```python
from build123d import *

# Parameters (mm, degrees)
SKETCH2_R           = 22.225
SKETCH2_R_2         = 19.05
SKETCH2_R_3         = 15.875
BOSS_EXTRUDE1_DEPTH = 3.175
SKETCH3_R           = 1.5875
BOSS_EXTRUDE2_DEPTH = 3.175
CUT_EXTRUDE1_DEPTH  = 3.175


with BuildPart() as part:
    # Sketch2 → Boss-Extrude1 (new body)
    with BuildSketch(Plane.XY):
        Circle(SKETCH2_R)
        Circle(SKETCH2_R_2, mode=Mode.SUBTRACT)
        Circle(SKETCH2_R_2)
        Circle(SKETCH2_R_3, mode=Mode.SUBTRACT)
    extrude(amount=BOSS_EXTRUDE1_DEPTH)

    # Sketch3 → Boss-Extrude2 (add)
    with BuildSketch(Plane.XY.offset(3.175)):
        with BuildLine():
            ThreePointArc((-16.148535057, 15.270083186), (-13.77482484, 17.441468562), (-11.1125, 19.247414599))
            Line((-11.1125, 19.247414599), (-17.4625, 30.245937227))
            Line((-17.4625, 30.245937227), (-22.961761314, 27.070937227))
            Line((-22.961761314, 27.070937227), (-16.611761314, 16.072414599))
            Line((-16.611761314, 16.072414599), (-16.148535057, 15.270083186))
        make_face()
        with Locations((-18.624630657, 25.90880657)):
            Circle(SKETCH3_R, mode=Mode.SUBTRACT)
        with BuildLine():
            Line((17.4625, 30.245937227), (11.1125, 19.247414599))
            ThreePointArc((11.1125, 19.247414599), (13.77482484, 17.441468562), (16.148535057, 15.270083186))
            Line((16.148535057, 15.270083186), (16.611761314, 16.072414599))
            Line((16.611761314, 16.072414599), (22.961761314, 27.070937227))
            Line((22.961761314, 27.070937227), (17.4625, 30.245937227))
        make_face()
        with Locations((18.624630657, 25.90880657)):
            Circle(SKETCH3_R, mode=Mode.SUBTRACT)
    extrude(amount=-BOSS_EXTRUDE2_DEPTH)

    # Sketch5 → Cut-Extrude1 (cut)
    with BuildSketch(Plane.XY.offset(3.175)):
        with BuildLine():
            Line((-11.1125, 19.247414599), (0, 0))
            Line((0, 0), (11.1125, 19.247414599))
            ThreePointArc((11.1125, 19.247414599), (0, 22.225), (-11.1125, 19.247414599))
        make_face()
    extrude(amount=-CUT_EXTRUDE1_DEPTH, mode=Mode.SUBTRACT)


solid = part.part
```
Could you check a few things on this model? Use its own coordinates, in mm. A direction names the side the tool comes from. Round coordinates to 2 decimals unless told otherwise and drop trailing zeros. Order: outer loops, then holes, each group sorted by start corner. A loop starts at its lowest first (then second) coordinate and runs counter-clockwise, first axis right, second up. Notation, with made-up numbers: M -27,-35.5 L -19,-35.5 A16 cw -19,-13.5 Z; hole C 24.5,57.5 d6. An arc over 180 degrees is marked long. One line per question, with ' | ' between items. Start each with the question number.
(1) Please list where these lines run through material, in increasing order: line 1 along X through (y, z) = (0, 1.95) (3 decimals); line 2 along Y through (x, z) = (18, 0.5); line 3 along X through (y, z) = (7, 2.3).
(2) Suppose I cut it at B-B on z = 1.75. Count the separate pieces of the cut face and the enclosed holes in it, then the cut area to 3 significant figures.
(3) For faces 1 (the face through (-12.633, 21.882, 1.61)), 2 (the face through (-20.174, 28.681, 1.61)), which set-ups out of +Z, -Z, +X, -X, +Y, -Y let a thin tool reach every point of the face, with its end or its side?
(4) For P1, Ø1, axis at y = -1, z = 1, coming from the +X side; P2, Ø1, axis at y = 7.5, z = 2.5, coming from the -X side, each with a flat end and sliding along its axis, tell me the tip position at first contact or that it passes through.
(5) Thinking about a two-plate mould opening in Y: for faces 3 (the face through (12.633, 21.882, 1.61)), 4 (the face through (-17.89, 24.5, 1.61)), 5 (the face through (-9, 14, 3.175)), 6 (the face through (19.36, 24.5, 1.61)), which applies, +Y half, -Y half, draft (parallel to the pull), parting line (faces both ways), or undercut?
(6) Suppose I cut it at C-C on x = 12. List the corners of the cut face in (y, z) for me (3 decimals), then the cut area to 3 significant figures.
(7) Suppose I cut it at A-A on y = 4. List the corners of the cut face in (x, z) for me (3 decimals), then the cut area to 3 significant figures.
(8) Suppose I cut it at D-D on x = 0. List the corners of the cut face in (y, z) for me (3 decimals).
Geometry results:
1) line 1: -22.225 to -15.875, 15.875 to 22.225 | line 2: -13.04 to 13.04, 18.48 to 24.45, 27.37 to 29.94 | line 3: -21.09 to -14.25, 14.25 to 21.09
2) separate pieces: 1 | enclosed holes: 2 | area: 783 mm²
3) face 1: +Z, -Z, +Y | face 2: +Z, -Z, -X, +Y
4) P1: x = 22.22 | P2: x = -21.09
5) face 3: +Y half | face 4: undercut | face 5: draft | face 6: undercut
6) outline: M -18.707,0 L -10.393,0 L -10.393,3.175 L -18.707,3.175 Z; M 10.393,0 L 20.785,0 L 20.785,3.175 L 10.393,3.175 Z | area: 59.4 mm²
7) outline: M -21.862,0 L -15.363,0 L -15.363,3.175 L -21.862,3.175 Z; M 15.363,0 L 21.862,0 L 21.862,3.175 L 15.363,3.175 Z | area: 41.3 mm²
8) outline: M -22.225,0 L -15.875,0 L -15.875,3.175 L -22.225,3.175 Z
